Read the model definition and answer for the solid it produces. Units are mm, in the model's axes. Face numbers are marked on the shaded views. Coordinates: 2 decimals unless noted, no trailing zeros. Write each loop counter-clockwise with the first axis right and the second up, starting at its lowest first coordinate (ties: lowest second). Pieces come first, ordered by that corner, then holes.
1) Find the intervals of material crossed by line 1 (Y direction, x = 3.81, z = -19); line 2 (Y direction, x = 4.5, z = -13.5); line 3 (Y direction, x = 2, z = -32), in increasing order.
2) Determine the mould class of the marked faces 1, 2 and 3 for opening direction Y: +Y half, -Y half, draft (parallel to the pull), parting line (faces both ways), or undercut.
3) The part is cut by section A-A (x = 3.81). Give the number of separate pieces and of enclosed holes in the cut face, then the cut area to 3 significant figures.
4) This flat-tipped pin is pushed along its axis until it touches: pin 1 Ø2.5 at (x, y) = (3.81, 9.525) entering from -Z. Where does it stop, or does it pass through?
5) The part is cut by section D-D (x = 6.75). Determine the outline of the cut face in (y, z) (3 decimals), then the cut area to 3 significant figures.
6) The part is cut by section B-B (z = -21.5). Determine the outline of the cut face in (x, y) (1 decimal), then the cut area to 3 significant figures.
7) The part is cut by section C-C (y = 19.05). Determine the outline of the cut face in (x, z).
Autodesk Inventor part; units mm, degrees
ref_plane "YZ Plane" through (0, 0, 0) normal (1, 0, 0) x (0, 1, 0)
ref_plane "XZ Plane" through (0, 0, 0) normal (0, 1, 0) x (-1, 0, 0)
ref_plane "XY Plane" through (0, 0, 0) normal (0, 0, 1) x (1, 0, 0)
sketch "Sketch1" plane through (0, 0, 0) normal (1, 0, 0) x (0, 1, 0)
  line L0 (0, 0) -> (38.1, 0)
  line L1 (38.1, 0) -> (38.1, -38.1)
  line L2 (38.1, -38.1) -> (0, -38.1)
  line L3 (0, -38.1) -> (0, 0)
  circle A0 centre (19.05, -19.05) radius 6.35
  dimension "d0" = 38.1
  dimension "d1" = 38.1
  dimension "d2" = 12.7
extrude "Extrusion1" add sketch "Sketch1" along normal blind 7.62
chamfer "Chamfer1" distance 3.175 angle 45 4 edges at (3.81, 38.1, 0) (3.81, 38.1, -38.1) (3.81, 0, 0) (3.81, 0, -38.1)
sketch "Sketch2" plane through (0, 3.175, -38.1) normal (0, 0, -1) x (-1, 0, 0)
  line L0 (0, 0) -> (-7.62, 0)
  line L1 (0, 31.75) -> (0, 0)
  line L2 (-7.62, 31.75) -> (0, 31.75)
  line L3 (-7.62, 0) -> (-7.62, 31.75)
  line L4 (-3.81, 15.875) -> (-3.81, 25.4)
  line L5 (-3.81, 25.4) -> (-3.81, 6.35)
  point P0 (0, -3.175)
  dimension "d10" = 9.525
  dimension "d11" = 19.05
hole "Hole1" at (3.81, 28.575, -38.1) at (3.81, 9.525, -38.1) direction (0, 0, 1) diameter 4.445 end through all
properties part number "1.5 in bearing block"
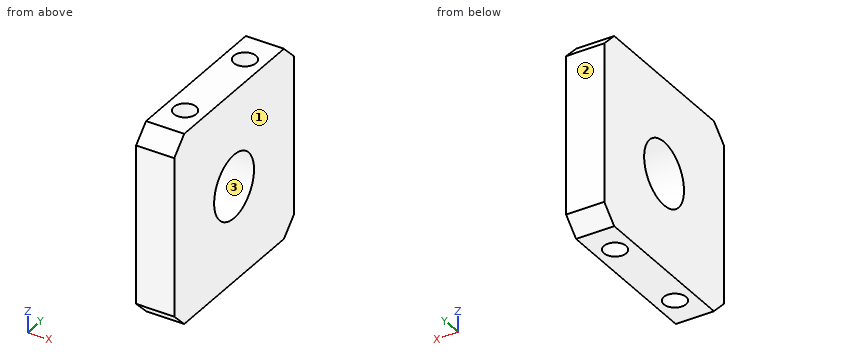
Reported:
1. line 1: y = 0 to 7.3, 11.75 to 12.7, 25.4 to 26.35, 30.8 to 38.1
1. line 2: y = 0 to 7.41, 11.64 to 15.96, 22.14 to 26.46, 30.69 to 38.1
1. line 3: y = 0 to 8.24, 10.81 to 27.29, 29.86 to 38.1
2. face 1: draft
2. face 2: +Y half
2. face 3: undercut
3. separate pieces: 3
3. enclosed holes: 1
3. area: 966 mm2
4. pin 1: passes through
5. outline: (0, -34.925) - (3.175, -38.1) - (34.925, -38.1) - (38.1, -34.925) - (38.1, -3.175) - (34.925, 0) - (3.175, 0) - (0, -3.175) - close; hole circle Ø12.7 at (19.05, -19.05)
5. area: 1,300 mm2
6. outline: (0, 0) - (7.6, 0) - (7.6, 13.2) - (0, 13.2) - close; (0, 24.9) - (7.6, 24.9) - (7.6, 38.1) - (0, 38.1) - close; hole circle Ø4.4 at (3.8, 9.5); hole circle Ø4.4 at (3.8, 28.6)
6. area: 170 mm2
7. outline: (0, -38.1) - (7.62, -38.1) - (7.62, -25.4) - (0, -25.4) - close; (0, -12.7) - (7.62, -12.7) - (7.62, 0) - (0, 0) - close
